Build history of the part. All positions in model axes, mm. A direction names the side the tool comes from. Give positions to 0.01 mm unless a question says otherwise; leave off trailing zeros. Order: outer loops, then holes, each group sorted by start corner. A loop starts at its lowest first (then second) coordinate and runs counter-clockwise, first axis right, second up. Notation, with made-up numbers: M -38,27.5 L -1,27.5 A13 ccw -1,31.5 Z; hole C 42,-16 d8. An arc over 180 degrees is marked long. Use CSV: the item, a comma, the result in double quotes. Start each with the question number.
Item 1: Wall check: line 1 along Z through (x, y) = (5, -65.85); line 2 along X through (y, z) = (-106.5, 10.5); line 3 along Z through (x, y) = (25.5, -85). Give the ranges that are in metal, low to high.
Item 2: Band-saw the part on B-B on y = -93.5. Give the number of separate pieces and of enclosed holes in the cut face, plus the area to 3 significant figures.
Item 3: Band-saw the part on D-D on z = -17. Write the cut outline in (x, y).
Item 4: Band-saw the part on A-A on z = 8.75. Write the cut outline in (x, y), plus the area to 3 significant figures.
Item 5: Pin check, flat tips, straight feed: P1, Ø0.6, axis at x = 39, z = -28, coming from the -Y side; P2, Ø3, axis at x = 5, z = -8, coming from the -Y side; P3, Ø12, axis at x = -8.5, y = -101.5, coming from the -Z side. Stop position of each tip, or through.
Item 6: Two-plate mould, pull along Y, no slides. Class faces 1 (the flat face through (38, -102, -2)), 2 (the flat face through (-1, -64.292, -8)), 3 (the cylindrical face through (22.905, -65.278, 9.229)), 4 (the cylindrical face through (0.5, -141, -0.5)): pulls with the +Y half, pulls with the -Y half, needs draft (parallel to the pull), parting line crosses it, or undercut.
Item 7: Band-saw the part on C-C on x = -11.75. Write the cut outline in (y, z).
Item 8: Which spindle directions (+Z, -Z, +X, -X, +Y, -Y) get a long thin tool onto all of the face, cutting with end or side? Do faces 5 (the flat face through (-38, -101, -2)), 6 (the flat face through (0.2, -141.4, -35)), 7 (the cylindrical face through (4.73, -65.28, 26.72)). Say none if no direction does.
from build123d import *

# Parameters (mm, degrees)
BOSS_EXTRUDE1_DEPTH     = 35
SHELL1_T                = -2
SKETCH3_R               = 15
SKETCH3_R_2             = 1.25
CUT_EXTRUDE2_DEPTH      = 2
SKETCH4_W               = 2.5
SKETCH4_H               = 40
CUT_EXTRUDE3_DEPTH      = 1
CUT_EXTRUDE3_DEPTH_BACK = 81
BOSS_EXTRUDE2_DEPTH     = 2


with BuildPart() as part:
    # Sketch1 → Boss-Extrude1 (new body, symmetric)
    with BuildSketch(Plane.XY):
        with BuildLine():
            Line((-40, -137.291660344), (-40, -64.291660344))
            Line((-40, -64.291660344), (40, -64.291660344))
            Line((40, -64.291660344), (40, -137.291660344))
            ThreePointArc((40, -137.291660344), (0, -143), (-40, -137.291660344))
        make_face()
    extrude(amount=BOSS_EXTRUDE1_DEPTH, both=True)

    # Shell1
    shell1_openings = [part.faces().sort_by_distance(p)[0] for p in [
        (0, -102.218745258, -35),
    ]]
    offset(amount=SHELL1_T, openings=shell1_openings, kind=Kind.INTERSECTION)

    # Sketch3 → Cut-Extrude2 (cut)
    with BuildSketch(Plane(origin=(0, -64.291660344, 0), x_dir=(1, 0, 0), z_dir=(0, 1, 0))):
        with Locations((5, -8.75)):
            Circle(SKETCH3_R)
        with Locations((5, 8)):
            Circle(SKETCH3_R_2)
        with Locations((21.75, -8.75)):
            Circle(SKETCH3_R_2)
        with Locations((-11.75, -8.75)):
            Circle(SKETCH3_R_2)
        with Locations((5, -25.5)):
            Circle(SKETCH3_R_2)
    extrude(amount=-CUT_EXTRUDE2_DEPTH, mode=Mode.SUBTRACT)

    # Sketch4 → Cut-Extrude3 (cut, two sides)
    with BuildSketch(Plane(origin=(40, 0, 0), x_dir=(0, 0, -1), z_dir=(1, 0, 0))) as cut_extrude3_sk:
        with Locations((24.25, -100.496660344)):
            Rectangle(SKETCH4_W, SKETCH4_H)
        with Locations((27.75, -100.496660344)):
            Rectangle(SKETCH4_W, SKETCH4_H)
        with Locations((31.25, -100.496660344)):
            Rectangle(SKETCH4_W, SKETCH4_H)
    extrude(amount=CUT_EXTRUDE3_DEPTH, mode=Mode.SUBTRACT)
    extrude(cut_extrude3_sk.sketch, amount=-CUT_EXTRUDE3_DEPTH_BACK, mode=Mode.SUBTRACT)

    # Sketch6 → Boss-Extrude2 (add)
    with BuildSketch(Plane(origin=(0, 0, -35), x_dir=(-1, 0, 0), z_dir=(0, 0, -1))):
        Polygon((-40, -64.291660344), (-40, -133.291660344), (-38, -133.291660344), (-38, -66.291660344), (38, -66.291660344), (38, -133.291660344), (40, -133.291660344), (40, -64.291660344), align=None)
    extrude(amount=BOSS_EXTRUDE2_DEPTH)


solid = part.part
Model answer:
1,line 1,"z = -37 to -9.25, -6.75 to -6.25, 23.75 to 24.25, 26.75 to 35"
1,line 2,"x = -40 to -38, 38 to 40"
1,line 3,"z = 33 to 35"
2,separate pieces,"7"
2,enclosed holes,"0"
2,area,"410 mm^2"
3,outline,"M -40,-137.29 A143 ccw 40,-137.29 L 40,-64.29 L -40,-64.29 Z; hole M -38,-135.78 A141 ccw 38,-135.78 L 38,-66.29 L -38,-66.29 Z"
4,outline,"M -40,-137.29 A143 ccw 40,-137.29 L 40,-64.29 L 23,-64.29 L 23,-66.29 L 38,-66.29 L 38,-135.78 A141 cw -38,-135.78 L -38,-66.29 L -13,-66.29 L -13,-64.29 L -40,-64.29 Z; M -10.5,-66.29 L -10,-66.29 L -10,-64.29 L -10.5,-64.29 Z; M 20,-66.29 L 20.5,-66.29 L 20.5,-64.29 L 20,-64.29 Z"
4,area,"529 mm^2"
5,P1,"stops at y = -137.66"
5,P2,"stops at y = -142.96"
5,P3,"stops at z = 33"
6,face 1,"undercut"
6,face 2,"pulls with the +Y half"
6,face 3,"needs draft"
6,face 4,"undercut"
7,outline,"M -142.52,-35 L -140.51,-35 L -140.51,33 L -66.29,33 L -66.29,10 L -64.29,10 L -64.29,35 L -142.52,35 Z; M -66.29,-37 L -64.29,-37 L -64.29,7.5 L -66.29,7.5 Z"
8,face 5,"-Z"
8,face 6,"-Z, +X, -X, -Y"
8,face 7,"+Y"
